Part model, mm, in its own coordinate system. A direction names the side the tool comes from. Give positions to 0.01 mm unless a question says otherwise; leave off trailing zeros. Write each loop counter-clockwise with the first axis right and the second up, starting at its lowest first coordinate (ties: lowest second). Pieces come first, ordered by that corner, then holes.
from build123d import *

# Parameters (mm, degrees)
F1_DEPTH = 400.05
F2_R     = 2.6162
F2_R_2   = 3.302
F3_DEPTH = 3.176


with BuildPart() as f1:
    # F0 (on Right) → F1 (new body)
    with BuildSketch(Plane.YZ):
        with BuildLine():
            Line((0, -44.45), (0, 0))
            Line((0, 0), (-3.175, 0))
            Line((-3.175, 0), (-3.175, -50.8))
            Line((-3.175, -50.8), (47.625, -50.8))
            Line((47.625, -50.8), (47.625, -47.625))
            Line((47.625, -47.625), (3.175, -47.625))
            ThreePointArc((3.175, -47.625), (0.929936, -46.695064), (0, -44.45))
        make_face()
    extrude(amount=-F1_DEPTH)

    # F2 (on face) → F3 (cut, through all)
    with BuildSketch(Plane(origin=(0, 0, 0), x_dir=(-1, 0, 0), z_dir=(0, 1, 0))):
        with Locations((9.525, -25.4)):
            Circle(F2_R)
        with Locations((390.525, -25.4)):
            Circle(F2_R)
        with Locations((159.5374, -25.4)):
            Circle(F2_R)
        with Locations((240.5126, -25.4)):
            Circle(F2_R)
        with Locations((223.0247, -25.4)):
            Circle(F2_R_2)
        with Locations((177.0253, -25.4)):
            Circle(F2_R_2)
        with Locations((249.5931, -7.9375)):
            Circle(F2_R)
        with Locations((150.4696, -7.9375)):
            Circle(F2_R)
    extrude(amount=-F3_DEPTH, mode=Mode.SUBTRACT)


solid = f1.part
1) Drill centre lines: L1, parallel to Y at x = -245, z = -20 (3 decimals); L2, parallel to Z at x = -338.5, y = 16.5 (3 decimals). Where is each one in solid material? Low to high.
Check result:
L1: y = -3.175 to 0
L2: z = -50.8 to -47.625
2) 3-axis set-ups, long thin cutter, end or side, ignore diameter. For faces 1 (the flat face through (-197, 26, -47.625)), 2 (the flat face through (0, -0.5, -36.6)): which of +Z, -Z, +X, -X, +Y, -Y reach the whole face in a straight line?
Check result:
face 1: +Z, +X, -X, +Y
face 2: +Z, -Z, +X, +Y, -Y
3) Flat gauge pins, fed straight in: P1, Ø3, axis at x = -269, z = -44, coming from the +Y side; P2, Ø7, axis at x = -150.47, z = -7.94, coming from the -Y side (3 decimals); P3, Ø8, axis at x = -230.5, z = -8, coming from the +Y side; P4, Ø6, axis at x = -177.03, z = -25.4, coming from the -Y side. Where does each tip first touch, or does it go through?
Check result:
P1: stops at y = 0.18
P2: stops at y = -3.175
P3: stops at y = 0
P4: passes through
4) Saw through at A-A (x = -234.5). Write the cut outline in (y, z) (3 decimals), and give its area (3 significant figures).
Check result:
outline: (-3.175, -50.8) - (47.625, -50.8) - (47.625, -47.625) - (3.175, -47.625) arc R3.175 cw to (0, -44.45) - (0, 0) - (-3.175, 0) - close
area: 315 mm2
5) Saw through at B-B (y = 31). Write the cut outline in (x, z) (3 decimals), and give its area (3 significant figures).
Check result:
outline: (-400.05, -50.8) - (0, -50.8) - (0, -47.625) - (-400.05, -47.625) - close
area: 1,270 mm2
6) Mould opens along Z. For faces 3 (the cylindrical face through (-173.726, -1.565, -25.255)), 4 (the flat face through (-400.05, -0.5, -36.6)), 5 (the flat face through (-197, 22, -50.8)) say: +Z half, -Z half, draft (parallel to the pull), parting line (faces both ways), or undercut.
Check result:
face 3: undercut
face 4: draft
face 5: -Z half
